from build123d import *

# Parameters (mm, degrees)
SKIZZE1_W                       = 20
SKIZZE1_H                       = 10
AUFSATZ_LINEAR_AUSTRAGEN1_DEPTH = 5
SCHNITT_LINEAR_AUSTRAGEN2_DEPTH = 2
VERRUNDUNG2_R                   = 0.5
VERRUNDUNG3_R                   = 0.5
VERRUNDUNG4_R                   = 0.5
VERRUNDUNG5_R                   = 0.5
VERRUNDUNG6_R                   = 0.5
VERRUNDUNG7_R                   = 0.5


with BuildPart() as part:
    # Skizze1 → Aufsatz-Linear austragen1 (new body)
    with BuildSketch(Plane.XY):
        with Locations((10, 5)):
            Rectangle(SKIZZE1_W, SKIZZE1_H)
    extrude(amount=AUFSATZ_LINEAR_AUSTRAGEN1_DEPTH)

    # Skizze3 → Schnitt-Linear austragen2 (cut)
    with BuildSketch(Plane.XY.offset(5)):
        with BuildLine():
            Line((4, 7), (16, 7))
            ThreePointArc((16, 7), (16.707106781, 6.707106781), (17, 6))
            Line((17, 6), (17, 4))
            ThreePointArc((17, 4), (16.707106781, 3.292893219), (16, 3))
            Line((16, 3), (4, 3))
            ThreePointArc((4, 3), (3.292893219, 3.292893219), (3, 4))
            Line((3, 4), (3, 6))
            ThreePointArc((3, 6), (3.292893219, 6.707106781), (4, 7))
        make_face()
    extrude(amount=-SCHNITT_LINEAR_AUSTRAGEN2_DEPTH, mode=Mode.SUBTRACT)

    # Verrundung2
    verrundung2_edges = [part.edges().sort_by_distance(p)[0] for p in [
        (3.292893219, 3.292893219, 5),
        (10, 3, 5),
        (16.707106781, 3.292893219, 5),
        (17, 5, 5),
        (16.707106781, 6.707106781, 5),
        (10, 7, 5),
        (3.292893219, 6.707106781, 5),
        (3, 5, 5),
    ]]
    fillet(verrundung2_edges, radius=VERRUNDUNG2_R)

    # Verrundung3
    verrundung3_edges = [part.edges().sort_by_distance(p)[0] for p in [
        (20, 5, 5),
        (10, 10, 5),
        (0, 5, 5),
        (10, 0, 5),
    ]]
    fillet(verrundung3_edges, radius=VERRUNDUNG3_R)

    # Verrundung4
    # the kernel refuses this fillet: 0.5 mm, written as the material it takes off along each edge
    with BuildSketch(Plane(origin=(19.5, 9.5, 4.5), x_dir=(0, 1, 0), z_dir=(1, 0, 0))) as verrundung4_piece_1_section:
        Polygon((0, 0), (VERRUNDUNG4_R, 0), (VERRUNDUNG4_R, VERRUNDUNG4_R), (0, VERRUNDUNG4_R), align=None)
    verrundung4_piece_1 = extrude(amount=VERRUNDUNG4_R, mode=Mode.PRIVATE)
    verrundung4_piece_1 = verrundung4_piece_1 - Plane(origin=(19.5, 9.5, 4.5), x_dir=(0, -0.7071067811865475, -0.7071067811865475), z_dir=(1, 0, 0)) * Sphere(VERRUNDUNG4_R, mode=Mode.PRIVATE)
    add(verrundung4_piece_1, mode=Mode.SUBTRACT)
    with BuildSketch(Plane(origin=(20, 10, -1.25), x_dir=(0, -1, 0), z_dir=(0, 0, 1))) as verrundung4_piece_2:
        with BuildLine():
            CenterArc((VERRUNDUNG4_R, -VERRUNDUNG4_R), VERRUNDUNG4_R, 90, 90)
            Line((0, -VERRUNDUNG4_R), (0, 0))
            Line((0, 0), (VERRUNDUNG4_R, 0))
        make_face()
    extrude(amount=5.75, mode=Mode.SUBTRACT)

    # Verrundung5
    # the kernel refuses this fillet: 0.5 mm, written as the material it takes off along each edge
    with BuildSketch(Plane(origin=(0.5, 9.5, 4.5), x_dir=(-1, 0, 0), z_dir=(0, 1, 0))) as verrundung5_piece_1_section:
        Polygon((0, 0), (VERRUNDUNG5_R, 0), (VERRUNDUNG5_R, VERRUNDUNG5_R), (0, VERRUNDUNG5_R), align=None)
    verrundung5_piece_1 = extrude(amount=VERRUNDUNG5_R, mode=Mode.PRIVATE)
    verrundung5_piece_1 = verrundung5_piece_1 - Plane(origin=(0.5, 9.5, 4.5), x_dir=(0.7071067811865475, 0, -0.7071067811865475), z_dir=(0, 1, 0)) * Sphere(VERRUNDUNG5_R, mode=Mode.PRIVATE)
    add(verrundung5_piece_1, mode=Mode.SUBTRACT)
    with BuildSketch(Plane(origin=(0, 10, -1.25), x_dir=(1, 0, 0), z_dir=(0, 0, 1))) as verrundung5_piece_2:
        with BuildLine():
            CenterArc((VERRUNDUNG5_R, -VERRUNDUNG5_R), VERRUNDUNG5_R, 90, 90)
            Line((0, -VERRUNDUNG5_R), (0, 0))
            Line((0, 0), (VERRUNDUNG5_R, 0))
        make_face()
    extrude(amount=5.75, mode=Mode.SUBTRACT)

    # Verrundung6
    # the kernel refuses this fillet: 0.5 mm, written as the material it takes off along each edge
    with BuildSketch(Plane(origin=(0.5, 0.5, 4.5), x_dir=(-1, 0, 0), z_dir=(0, -1, 0))) as verrundung6_piece_1_section:
        Polygon((0, 0), (VERRUNDUNG6_R, 0), (VERRUNDUNG6_R, -VERRUNDUNG6_R), (0, -VERRUNDUNG6_R), align=None)
    verrundung6_piece_1 = extrude(amount=VERRUNDUNG6_R, mode=Mode.PRIVATE)
    verrundung6_piece_1 = verrundung6_piece_1 - Plane(origin=(0.5, 0.5, 4.5), x_dir=(0.7071067811865475, 0, -0.7071067811865475), z_dir=(0, -1, 0)) * Sphere(VERRUNDUNG6_R, mode=Mode.PRIVATE)
    add(verrundung6_piece_1, mode=Mode.SUBTRACT)
    with BuildSketch(Plane(origin=(0, 0, -1.25), x_dir=(1, 0, 0), z_dir=(0, 0, 1))) as verrundung6_piece_2:
        with BuildLine():
            CenterArc((VERRUNDUNG6_R, VERRUNDUNG6_R), VERRUNDUNG6_R, 180, 90)
            Line((0, VERRUNDUNG6_R), (0, 0))
            Line((0, 0), (VERRUNDUNG6_R, 0))
        make_face()
    extrude(amount=5.75, mode=Mode.SUBTRACT)

    # Verrundung7
    # the kernel refuses this fillet: 0.5 mm, written as the material it takes off along each edge
    with BuildSketch(Plane(origin=(19.5, 0.5, 4.5), x_dir=(0, -1, 0), z_dir=(1, 0, 0))) as verrundung7_piece_1_section:
        Polygon((0, 0), (VERRUNDUNG7_R, 0), (VERRUNDUNG7_R, -VERRUNDUNG7_R), (0, -VERRUNDUNG7_R), align=None)
    verrundung7_piece_1 = extrude(amount=VERRUNDUNG7_R, mode=Mode.PRIVATE)
    verrundung7_piece_1 = verrundung7_piece_1 - Plane(origin=(19.5, 0.5, 4.5), x_dir=(0, 0.7071067811865475, -0.7071067811865475), z_dir=(1, 0, 0)) * Sphere(VERRUNDUNG7_R, mode=Mode.PRIVATE)
    add(verrundung7_piece_1, mode=Mode.SUBTRACT)
    with BuildSketch(Plane(origin=(20, 0, -1.25), x_dir=(0, 1, 0), z_dir=(0, 0, 1))) as verrundung7_piece_2:
        with BuildLine():
            CenterArc((VERRUNDUNG7_R, VERRUNDUNG7_R), VERRUNDUNG7_R, 180, 90)
            Line((0, VERRUNDUNG7_R), (0, 0))
            Line((0, 0), (VERRUNDUNG7_R, 0))
        make_face()
    extrude(amount=5.75, mode=Mode.SUBTRACT)


solid = part.part
Model file for the job. Use its own axes, mm. A direction names the side the tool comes from. Coordinates: 2 decimals unless noted, no trailing zeros. Order: outer loops, then holes, each group sorted by start corner. A loop starts at its lowest first (then second) coordinate and runs counter-clockwise, first axis right, second up. Notation, with made-up numbers: (-17, 1) -> (22, 1) arc R24 ccw to (22, 15) -> close; hole circle Ø11 at (-5.5, -1.75). An arc over 180 degrees is marked (long way). Return JSON: item names as keys, results as strings. Group by question number.
Item 1: Saw through at A-A on z = 4.1. Write the cut outline in (x, y).
Item 2: Tool access for faces 5 (the flat face through (10, 0, 2)), 6 (the flat face through (10, 3, 4)): list every direction of +Z, -Z, +X, -X, +Y, -Y with a clear straight run to the whole face (end or side of a thin tool).
Item 3: Wall check: line 1 along Y through (x, z) = (12.25, 4.5); line 2 along Z through (x, y) = (16.5, 6.25); line 3 along X through (y, z) = (3.5, 4.2). Give the ranges that are in metal, low to high. Write a range as [from, to].
Item 4: Pull direction X, two halves, no side cores. Call faces 1 (the flat face through (10, 10, 2)), 2 (the flat face through (0, 5, 2)), 3 (the cylindrical face through (16.699, 6.715, 3.76)), 4 (the cylindrical face through (3.285, 6.699, 3.76)): pulls with the +X half, pulls with the -X half, needs draft (parallel to the pull), parting line crosses it, or undercut.
Item 5: Flat gauge pin, fed straight in: P1, Ø2, axis at x = 15, z = 1.5, coming from the -Y side. Where does the tip first touch, or does it go through?
Item 6: Saw through at B-B on y = 4.25. Write the cut outline in (x, z), then the cut area to 3 significant figures.
Item 7: Saw through at C-C on x = 12. Write the cut outline in (y, z).
Values found:
{
 "1": {"outline": "(0, 0.5) arc R0.5 ccw to (0.5, 0) -> (19.5, 0) arc R0.5 ccw to (20, 0.5) -> (20, 9.5) arc R0.5 ccw to (19.5, 10) -> (0.5, 10) arc R0.5 ccw to (0, 9.5) -> close; hole (3, 4) arc R1 ccw to (4, 3) -> (16, 3) arc R1 ccw to (17, 4) -> (17, 6) arc R1 ccw to (16, 7) -> (4, 7) arc R1 ccw to (3, 6) -> close"},
 "2": {"face 5": "+Z, -Z, +X, -X, -Y", "face 6": "+Z"},
 "3": {"line 1": "y = [0, 3], [7, 10]", "line 2": "z = [0, 3]", "line 3": "x = [0, 3.13], [16.87, 20]"},
 "4": {"face 1": "needs draft", "face 2": "pulls with the -X half", "face 3": "undercut", "face 4": "undercut"},
 "5": {"P1": "stops at y = 0"},
 "6": {"outline": "(0, 0) -> (20, 0) -> (20, 4.5) arc R0.5 ccw to (19.5, 5) -> (17.5, 5) arc R0.5 ccw to (17, 4.5) -> (17, 3) -> (3, 3) -> (3, 4.5) arc R0.5 ccw to (2.5, 5) -> (0.5, 5) arc R0.5 ccw to (0, 4.5) -> close", "area": "71.8 mm2"},
 "7": {"outline": "(0, 0) -> (10, 0) -> (10, 4.5) arc R0.5 ccw to (9.5, 5) -> (7.5, 5) arc R0.5 ccw to (7, 4.5) -> (7, 3) -> (3, 3) -> (3, 4.5) arc R0.5 ccw to (2.5, 5) -> (0.5, 5) arc R0.5 ccw to (0, 4.5) -> close"}
}
